```python
from build123d import *

# Parameters (mm, degrees)
F0_W     = 711.2
F0_H     = 25.4
F1_DEPTH = 25.4
F2_W     = 19.05
F2_H     = 44.45
F3_DEPTH = 711.201
F4_R     = 2.4892
F5_DEPTH = 50.801
F6_R     = 2.4892
F7_DEPTH = 25.401


with BuildPart() as f1:
    # F0 (on Top) → F1 (new body, symmetric)
    with BuildSketch(Plane.XY):
        Rectangle(F0_W, F0_H)
    extrude(amount=F1_DEPTH, both=True)

    # F2 (on face) → F3 (cut, through all)
    with BuildSketch(Plane.YZ.offset(355.6)):
        Rectangle(F2_W, F2_H)
    extrude(amount=-F3_DEPTH, mode=Mode.SUBTRACT)

    # F4 (on face) → F5 (cut, through all)
    with BuildSketch(Plane.XY.offset(25.4)):
        with Locations((-342.9, 0)):
            Circle(F4_R)
        with Locations((-317.5, 0)):
            Circle(F4_R)
        with Locations((-292.1, 0)):
            Circle(F4_R)
        with Locations((-266.7, 0)):
            Circle(F4_R)
        with Locations((-241.3, 0)):
            Circle(F4_R)
        with Locations((-215.9, 0)):
            Circle(F4_R)
        with Locations((-190.5, 0)):
            Circle(F4_R)
        with Locations((-165.1, 0)):
            Circle(F4_R)
        with Locations((-139.7, 0)):
            Circle(F4_R)
        with Locations((-114.3, 0)):
            Circle(F4_R)
        with Locations((-88.9, 0)):
            Circle(F4_R)
        with Locations((-63.5, 0)):
            Circle(F4_R)
        with Locations((-38.1, 0)):
            Circle(F4_R)
        with Locations((-12.7, 0)):
            Circle(F4_R)
        with Locations((12.7, 0)):
            Circle(F4_R)
        with Locations((38.1, 0)):
            Circle(F4_R)
        with Locations((63.5, 0)):
            Circle(F4_R)
        with Locations((88.9, 0)):
            Circle(F4_R)
        with Locations((114.3, 0)):
            Circle(F4_R)
        with Locations((139.7, 0)):
            Circle(F4_R)
        with Locations((165.1, 0)):
            Circle(F4_R)
        with Locations((190.5, 0)):
            Circle(F4_R)
        with Locations((215.9, 0)):
            Circle(F4_R)
        with Locations((241.3, 0)):
            Circle(F4_R)
        with Locations((266.7, 0)):
            Circle(F4_R)
        with Locations((292.1, 0)):
            Circle(F4_R)
        with Locations((317.5, 0)):
            Circle(F4_R)
        with Locations((342.9, 0)):
            Circle(F4_R)
        with Locations((368.3, 0)):
            Circle(F4_R)
        with Locations((393.7, 0)):
            Circle(F4_R)
    extrude(amount=-F5_DEPTH, mode=Mode.SUBTRACT)

    # F6 (on face) → F7 (cut, through all)
    with BuildSketch(Plane.XZ.offset(12.7)):
        with BuildLine():
            ThreePointArc((-323.85, -15.875), (-321.990128, -20.365128), (-317.5, -22.225))
            Line((-317.5, -22.225), (-266.7, -22.225))
            ThreePointArc((-266.7, -22.225), (-262.209872, -20.365128), (-260.35, -15.875))
            Line((-260.35, -15.875), (-260.35, 15.875))
            ThreePointArc((-260.35, 15.875), (-262.209872, 20.365128), (-266.7, 22.225))
            Line((-266.7, 22.225), (-317.5, 22.225))
            ThreePointArc((-317.5, 22.225), (-321.990128, 20.365128), (-323.85, 15.875))
            Line((-323.85, 15.875), (-323.85, -15.875))
        make_face()
        with BuildLine():
            Line((317.5, 22.225), (266.7, 22.225))
            ThreePointArc((266.7, 22.225), (262.209872, 20.365128), (260.35, 15.875))
            Line((260.35, 15.875), (260.35, -15.875))
            ThreePointArc((260.35, -15.875), (262.209872, -20.365128), (266.7, -22.225))
            Line((266.7, -22.225), (317.5, -22.225))
            ThreePointArc((317.5, -22.225), (321.990128, -20.365128), (323.85, -15.875))
            Line((323.85, -15.875), (323.85, 15.875))
            ThreePointArc((323.85, 15.875), (321.990128, 20.365128), (317.5, 22.225))
        make_face()
        with BuildLine():
            Line((-19.05, 0), (19.05, 0))
            ThreePointArc((19.05, 0), (0, 19.05), (-19.05, 0))
        make_face()
        with Locations((-23.8125, 0)):
            Circle(F6_R)
        with BuildLine():
            ThreePointArc((-19.05, 0), (0, -19.05), (19.05, 0))
            Line((19.05, 0), (-19.05, 0))
        make_face()
        with BuildLine():
            ThreePointArc((26.3017, 0), (23.8125, 2.4892), (21.3233, 0))
            ThreePointArc((21.3233, 0), (23.8125, -2.4892), (26.3017, 0))
        make_face()
        with Locations((-57.15, 0)):
            Circle(F6_R)
        with Locations((57.15, 0)):
            Circle(F6_R)
    extrude(amount=-F7_DEPTH, mode=Mode.SUBTRACT)


solid = f1.part
```
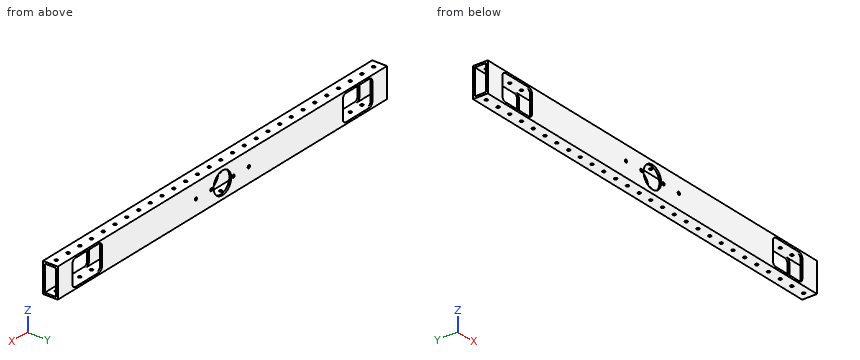
Build history of the part. All positions in model axes, mm. Round coordinates to 2 decimals unless told otherwise and drop trailing zeros. Order: outer loops, then holes, each group sorted by start corner. A loop starts at its lowest first (then second) coordinate and runs counter-clockwise, first axis right, second up. Notation, with made-up numbers: (49, 59.25) - (95, 59.25) arc R22 cw to (95, 82.25) - close; hole circle Ø7 at (46.25, 18.5). An arc over 180 degrees is marked (long way). Use a Markdown table: item, result.
1) Wall check: L1, parallel to Y at x = -39, z = 2 (3 decimals); L2, parallel to Z at x = -244.5, y = -4 (3 decimals); L3, parallel to Y at x = 215.9, z = 23.55. Give the ranges that are in metal, low to high.
Recorded:
| item | result |
|---|---|
| L1 | y = -12.7 to -9.525, 9.525 to 12.7 |
| L2 | z = -25.4 to -22.225, 22.225 to 25.4 |
| L3 | y = -12.7 to -2.49, 2.49 to 12.7 |
2) Saw through at A-A on x = 152. Write the cut outline in (y, z) (3 decimals), and give its area (3 significant figures).
Recorded:
| item | result |
|---|---|
| outline | (-12.7, -25.4) - (12.7, -25.4) - (12.7, 25.4) - (-12.7, 25.4) - close; hole (-9.525, -22.225) - (9.525, -22.225) - (9.525, 22.225) - (-9.525, 22.225) - close |
| area | 444 mm² |
3) Flat gauge pins, fed straight in: pin 1 Ø6.5 at (x, y) = (114.3, 0) entering from +Z; pin 2 Ø4.5 at (x, y) = (-165.1, 0) entering from -Z. Where does each tip first touch, or does it go through?
Recorded:
| item | result |
|---|---|
| pin 1 | stops at z = 25.4 |
| pin 2 | passes through |
4) Saw through at B-B on x = -308. Write the cut outline in (y, z) (3 decimals), and give its area (3 significant figures).
Recorded:
| item | result |
|---|---|
| outline | (-12.7, -25.4) - (12.7, -25.4) - (12.7, -22.225) - (-12.7, -22.225) - close; (-12.7, 22.225) - (12.7, 22.225) - (12.7, 25.4) - (-12.7, 25.4) - close |
| area | 161 mm² |
